Study the drawing (mm; zero at the part's minimum x, y, z) and answer. A direction names the side the tool comes from. Give positions to 0.01 mm unless a question says otherwise; leave off trailing zeros. Order: outer loops, then holes, each group sorted by start corner. A loop starts at its lowest first (then second) coordinate and runs counter-clockwise, first axis right, second up. Notation, with made-up numbers: (48, 79) - (66, 79) arc R22 cw to (66, 95) - close; hole circle Ø4 at (-38.75, 67). An arc over 180 degrees is marked (long way). Write each question's results on one line, items separated by ' | '. Start each with the question number.
1. Section A-A (x = 19) is taken. Give the vertices of the cut face in (y, z), and give its area (3 significant figures).
2. Determine the mould class of the marked faces 3, 4 and 5 for opening direction Y: released by +Y, released by -Y, zero draft, split by the parting line, or undercut.
3. Flat-ended cylindrical pins translate along their axes: pin 1 (3 mm diameter, centred on y = 18, z = 7, fed in from -X); pin 2 (0.6 mm diameter, centred on y = 16, z = 0.5, fed in from -X); pin 3 (1 mm diameter, centred on x = 7.5, y = 3, fed in from -Z). Find the tip coordinate at first contact, or state that the pin passes through.
4. Section C-C (y = 16.25) is taken. Give the vertices of the cut face in (x, z), and give its area (4 significant figures).
5. Which of the six approach directions +Z, -Z, +X, -X, +Y, -Y give full straight-line access (tool end or side, diameter ignored) to the marked faces 1 and 2?
6. Find the intervals of material crossed by L1, parallel to Y at x = 4, z = 10; L2, parallel to Z at x = 17.5, y = 9.25; L3, parallel to X at y = 4.75, z = 8, in increasing order.
7. Section B-B (z = 23.5) is taken. Give the vertices of the cut face in (x, y).
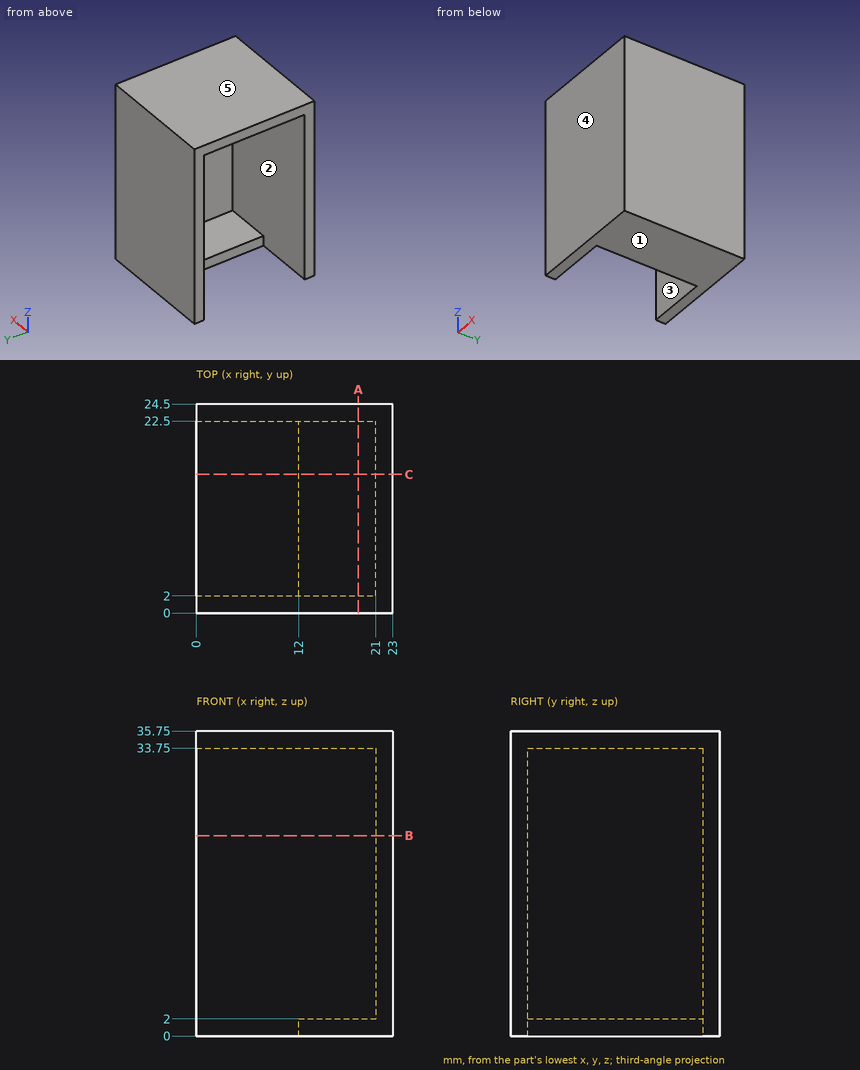
Reported:
1) outline: (0, 0) - (24.5, 0) - (24.5, 35.75) - (0, 35.75) - close; hole (2, 2) - (22.5, 2) - (22.5, 33.75) - (2, 33.75) - close | area: 225 mm²
2) face 3: undercut | face 4: released by -Y | face 5: zero draft
3) pin 1: x = 21 | pin 2: x = 12 | pin 3: z = 33.75
4) outline: (0, 33.75) - (21, 33.75) - (21, 2) - (12, 2) - (12, 0) - (23, 0) - (23, 35.75) - (0, 35.75) - close | area: 131.5 mm²
5) face 1: -Z, +X, -X, +Y, -Y | face 2: -X
6) L1: 0 to 2, 22.5 to 24.5 | L2: 0 to 2, 33.75 to 35.75 | L3: 21 to 23
7) outline: (0, 0) - (23, 0) - (23, 24.5) - (0, 24.5) - (0, 22.5) - (21, 22.5) - (21, 2) - (0, 2) - close
